Geometry: final body of the model. Coordinates: model frame, mm. A direction names the side the tool comes from. Give positions to 0.01 mm unless a question says otherwise; leave off trailing zeros. Write each loop counter-clockwise with the first axis right and the second up, starting at its lowest first coordinate (ties: lowest second). Pieces come first, ordered by that corner, then holes. Notation, with made-up numbers: M 54.5,42.25 L 101.5,42.25 A11 cw 101.5,46.25 Z; hole C 49,69 d7. An arc over 180 degrees is marked long. Use a Markdown table: item, result. Add a question column.
1) Set-up query: faces 4 (the flat face through (-697.5, -10, 39)), 5 (the flat face through (-767.5, -11, 39)), 6 (the flat face through (-10, 10, -21.696)). Return all of +Z, -Z, +X, -X, +Y, -Y with unobstructed straight access to the full face (end or side cutting, diameter ignored); none if empty.
2) Pin query (flat end, axial travel): pin 1 (10 mm diameter, centred on x = -420.5, y = -265, fed in from -Z); pin 2 (3 mm diameter, centred on y = 407, z = -14, fed in from +X); pin 3 (1.5 mm diameter, centred on x = -424, y = 428, fed in from +Z). Return the tip coordinate at first contact, or that it passes through.
3) Section A-A on z = 29. Return the cut outline in (x, y).
4) Draft query along Y for faces 1 (the flat face through (-60, -735, 80)), 2 (the flat face through (-11, -767.5, 39)), 3 (the flat face through (-10, 697.5, 39)). Return one class per face: +Y half, -Y half, draft (parallel to the pull), parting line (faces both ways), or undercut.
5) Line query: line 1 (Y direction, x = -324.5, z = 62); line 2 (Z direction, x = -89, y = 515.5). Output: solid intervals per line, ascending.
```python
from build123d import *

# Parameters (mm, degrees)
F0_W        = 1535
F0_H        = 1535
F0_W_2      = 1395
F0_H_2      = 1395
F1_DEPTH    = 80
F1_FACE_W   = 1535
F1_FACE_H   = 1535
F1_FACE_W_2 = 1395
F1_FACE_H_2 = 1395
F2_DEPTH    = 115
F2_TAPER    = 54.3
F3_W        = 1467.787861824
F3_H        = 1458.398938179
F4_DEPTH    = 21.696


with BuildPart() as f1:
    # F0 (on Top) → F1 (new body)
    with BuildSketch(Plane.XY):
        Rectangle(F0_W, F0_H)
        Rectangle(F0_W_2, F0_H_2, mode=Mode.SUBTRACT)
    extrude(amount=F1_DEPTH)

    # F1_face (on face) → F2 (join)
    with BuildSketch(Plane(origin=(0, 0, 0), x_dir=(1, 0, 0), z_dir=(0, 0, -1))):
        Rectangle(F1_FACE_W, F1_FACE_H)
        Rectangle(F1_FACE_W_2, F1_FACE_H_2, mode=Mode.SUBTRACT)
    extrude(amount=F2_DEPTH, taper=F2_TAPER)

    # F3 (on Top) → F4 (join)
    with BuildSketch(Plane.XY):
        Rectangle(F3_W, F3_H)
    extrude(amount=-F4_DEPTH)


solid = f1.part
```
Found:
| question | item | result |
|---|---|---|
| 1 | face 4 | +Z |
| 1 | face 5 | +Z, -Z, -X, +Y, -Y |
| 1 | face 6 | -Z |
| 2 | pin 1 | z = -21.7 |
| 2 | pin 2 | x = 750.1 |
| 2 | pin 3 | z = 0 |
| 3 | outline | M -767.5,-767.5 L 767.5,-767.5 L 767.5,767.5 L -767.5,767.5 Z; hole M -697.5,-697.5 L 697.5,-697.5 L 697.5,697.5 L -697.5,697.5 Z |
| 4 | face 1 | draft |
| 4 | face 2 | -Y half |
| 4 | face 3 | undercut |
| 5 | line 1 | -767.5 to -697.5, 697.5 to 767.5 |
| 5 | line 2 | -21.7 to 0 |
